```python
from build123d import *

# Parameters (mm, degrees)
F0_W      = 1.1809540468
F0_H      = 55.4866959378
F0_W_2    = 1.0430663562
F0_H_2    = 55.8827305807
F0_W_3    = 1.2505598919
F0_H_3    = 59.9420672474
F1_DEPTH  = 25.4
F2_DEPTH  = 19.05
F4_R      = 25.4
F5_R      = 12.7
F6_DEPTH  = 61.6204
F7_DEPTH  = 45.466
F8_DEPTH  = 87.0204
F10_DEPTH = 37.285599403


with BuildPart() as f1:
    # F0 (on Top) → F1 (new body)
    with BuildSketch(Plane.XY):
        with BuildLine():
            ThreePointArc((-31.4129105711, -45.2980363816), (-30.4781671858, -42.3561098061), (-30.1620009138, -39.2854883608))
            ThreePointArc((-30.1620009138, -39.2854883608), (-29.8463674498, -42.3560514479), (-28.912179671, -45.2980363816))
            Line((-28.912179671, -45.2980363816), (-12.330923231, -45.2980363816))
            Line((-12.330923231, -45.2980363816), (-1.2493222605, -45.2980363816))
            ThreePointArc((-1.2493222605, -45.2980363816), (-0.3153893091, -42.3572770972), (0.0004989823, -39.2879920805))
            Line((0.0004989823, -39.2879920805), (0, -47.9196608067))
            ThreePointArc((0, -47.9196608067), (0.6558623791, -52.3187849866), (2.5664044493, -56.3352857035))
            Line((2.5664044493, -56.3352857035), (27.5960955507, -56.3352857035))
            ThreePointArc((27.5960955507, -56.3352857035), (29.5066376209, -52.3187849866), (30.1625, -47.9196608067))
            Line((30.1625, -47.9196608067), (30.1656608492, -43.188519241))
            ThreePointArc((30.1656608492, -43.188519241), (30.9988064443, -48.131759315), (33.4061909682, -52.5288326332))
            Line((33.4061909682, -52.5288326332), (57.0876307301, -52.5288326332))
            ThreePointArc((57.0876307301, -52.5288326332), (59.4950152541, -48.131759315), (60.3281608492, -43.188519241))
            Line((60.3281608492, -43.188519241), (60.3281608492, 25.6428197026))
            ThreePointArc((60.3281608492, 25.6428197026), (46.2008131527, 40.6938718904), (30.2863311656, 27.5468042333))
            ThreePointArc((30.2863311656, 27.5468042333), (15.0360783361, 42.4746485662), (0, 27.3310989141))
            Line((0, 27.3310989141), (0, 31.4158573747))
            ThreePointArc((0, 31.4158573747), (-15.0810004563, 46.496857831), (-30.1620009126, 31.4158573747))
            Line((-30.1620009126, 31.4158573747), (-30.1620009127, 26.0546095664))
            ThreePointArc((-30.1620009127, 26.0546095664), (-45.243250861, 41.1358595153), (-60.3245008099, 26.0546095669))
            Line((-60.3245008099, 26.0546095669), (-60.3245008099, 0))
            Line((-60.3245008099, 0), (-60.3245008099, -39.2829846411))
            ThreePointArc((-60.3245008099, -39.2829846411), (-60.0085894761, -42.3548841799), (-59.0735911526, -45.2980363816))
            Line((-59.0735911526, -45.2980363816), (-31.4129105711, -45.2980363816))
        make_face()
        with Locations((-30.1620009133, -10.8462562301)):
            Rectangle(F0_W, F0_H, mode=Mode.SUBTRACT)
        with Locations((0.0002494911, -11.0644246154)):
            Rectangle(F0_W_2, F0_H_2, mode=Mode.SUBTRACT)
        with Locations((30.1857188067, -13.1142732591)):
            Rectangle(F0_W_3, F0_H_3, mode=Mode.SUBTRACT)
    extrude(amount=F1_DEPTH)

    # F0 (on Top) → F2 (join)
    with BuildSketch(Plane.XY):
        with BuildLine():
            ThreePointArc((-28.912179671, -45.2980363816), (-29.8463674498, -42.3560514479), (-30.1620009138, -39.2854883608))
            ThreePointArc((-30.1620009138, -39.2854883608), (-30.4781671858, -42.3561098061), (-31.4129105711, -45.2980363816))
            Line((-31.4129105711, -45.2980363816), (-59.0735911526, -45.2980363816))
            ThreePointArc((-59.0735911526, -45.2980363816), (-60.0085894761, -42.3548841799), (-60.3245008099, -39.2829846411))
            Line((-60.3245008099, -39.2829846411), (-60.3245008099, 0))
            Line((-60.3245008099, 0), (-70.1869130135, -37.5586524606))
            Line((-70.1869130135, -37.5586524606), (-70.1869130135, -49.070879817))
            Line((-70.1869130135, -49.070879817), (-63.4611696021, -73.2465684414))
            Line((-63.4611696021, -73.2465684414), (-12.330923231, -73.2465684414))
            ThreePointArc((-12.330923231, -73.2465684414), (1.6433427989, -59.2723024115), (-12.330923231, -45.2980363816))
            Line((-12.330923231, -45.2980363816), (-28.912179671, -45.2980363816))
        make_face()
    extrude(amount=F2_DEPTH)

    # F4
    f4_edges = [f1.edges().sort_by_distance(p)[0] for p in [
        (-70.186913, -37.558652, 9.525),
        (-70.186913, -49.07088, 9.525),
    ]]
    fillet(f4_edges, radius=F4_R)

    # F5
    f5_edges = [f1.edges().sort_by_distance(p)[0] for p in [
        (-63.46117, -73.246568, 9.525),
    ]]
    fillet(f5_edges, radius=F5_R)

    # F3 (on face) → F6 (join)
    with BuildSketch(Plane.XY):
        with BuildLine():
            Line((-30.7524779367, -35.9619690384), (-39.3256613186, -35.9619690384))
            Line((-39.3256613186, -35.9619690384), (-39.3256613186, -42.5913690384))
            Line((-39.3256613186, -42.5913690384), (-30.529074842, -42.5913690384))
            ThreePointArc((-30.529074842, -42.5913690384), (-30.2541193355, -40.9485795087), (-30.1620009138, -39.2854883608))
            ThreePointArc((-30.1620009138, -39.2854883608), (-30.0701620308, -40.9485637633), (-29.7954894935, -42.5913690384))
            Line((-29.7954894935, -42.5913690384), (-0.366012438, -42.5913690384))
            ThreePointArc((-0.366012438, -42.5913690384), (-0.0914778965, -40.9498079941), (0.0004989823, -39.2879920805))
            Line((0.0004989823, -39.2879920805), (0.0003080196, -42.5913690384))
            Line((0.0003080196, -42.5913690384), (29.4575386814, -42.5913690384))
            Line((29.4575386814, -42.5913690384), (29.4575386814, -35.9619690384))
            Line((29.4575386814, -35.9619690384), (0.5217826692, -35.9619690384))
            Line((0.5217826692, -35.9619690384), (0.5217826692, -39.0057899058))
            Line((0.5217826692, -39.0057899058), (-0.5212836869, -39.0057899058))
            Line((-0.5212836869, -39.0057899058), (-0.5212836869, -35.9619690384))
            Line((-0.5212836869, -35.9619690384), (-29.5715238899, -35.9619690384))
            Line((-29.5715238899, -35.9619690384), (-29.5715238899, -38.5896041989))
            Line((-29.5715238899, -38.5896041989), (-30.7524779367, -38.5896041989))
            Line((-30.7524779367, -38.5896041989), (-30.7524779367, -35.9619690384))
        make_face()
    extrude(amount=-F6_DEPTH)

    # F7 (add): a face of the model
    f7_faces = [f1.faces().sort_by_distance(p)[0] for p in [
        (-39.3256613186, -39.2766690384, -30.8102),
    ]]
    extrude(f7_faces, amount=-F7_DEPTH)

    # F8 (add, through all): a face of the model
    f8_faces = [f1.faces().sort_by_distance(p)[0] for p in [
        (-4.9340613186, -39.2766690384, -61.6204),
    ]]
    extrude(f8_faces, amount=-F8_DEPTH)

    # F9 (on face) → F10 (cut, through all)
    with BuildSketch(Plane(origin=(0, -35.9619690384, 0), x_dir=(-1, 0, 0), z_dir=(0, 1, 0))):
        with BuildLine():
            ThreePointArc((-23.3615386814, -50.546), (-25.2030386814, -48.7045), (-27.0445386814, -50.546))
            Line((-27.0445386814, -50.546), (-23.3615386814, -50.546))
        make_face()
        with BuildLine():
            Line((-23.3615386814, -50.546), (-27.0445386814, -50.546))
            ThreePointArc((-27.0445386814, -50.546), (-25.2030386814, -52.3875), (-23.3615386814, -50.546))
        make_face()
        with BuildLine():
            Line((-7.1055386814, -50.546), (-3.4225386814, -50.546))
            ThreePointArc((-3.4225386814, -50.546), (-5.2640386814, -48.7045), (-7.1055386814, -50.546))
        make_face()
        with BuildLine():
            ThreePointArc((-7.1055386814, -50.546), (-5.2640386814, -52.3875), (-3.4225386814, -50.546))
            Line((-3.4225386814, -50.546), (-7.1055386814, -50.546))
        make_face()
        with BuildLine():
            Line((13.2906613186, -50.546), (16.9736613186, -50.546))
            ThreePointArc((16.9736613186, -50.546), (15.1321613186, -48.7045), (13.2906613186, -50.546))
        make_face()
        with BuildLine():
            ThreePointArc((13.2906613186, -50.546), (15.1321613186, -52.3875), (16.9736613186, -50.546))
            Line((16.9736613186, -50.546), (13.2906613186, -50.546))
        make_face()
        with BuildLine():
            Line((33.2296613186, -50.546), (36.9126613186, -50.546))
            ThreePointArc((36.9126613186, -50.546), (35.0711613186, -48.7045), (33.2296613186, -50.546))
        make_face()
        with BuildLine():
            ThreePointArc((33.2296613186, -50.546), (35.0711613186, -52.3875), (36.9126613186, -50.546))
            Line((36.9126613186, -50.546), (33.2296613186, -50.546))
        make_face()
    extrude(amount=-F10_DEPTH, mode=Mode.SUBTRACT)


solid = f1.part
```
Can you work these out from the model? Positions are in its coordinate system, mm. A direction names the side the tool comes from. Coordinates: 2 decimals unless noted, no trailing zeros. Write each loop counter-clockwise with the first axis right and the second up, starting at its lowest first coordinate (ties: lowest second). Pieces come first, ordered by that corner, then holes. Notation, with made-up numbers: (-29.75, 25.25) - (0.25, 25.25) arc R20 ccw to (0.25, 60.25) - close; hole circle Ø11 at (63, 59). An arc over 180 degrees is marked (long way). Return JSON: item names as keys, results as strings.
Q1. If we section it at C-C (x = -23): Please give me the cut outline in (y, z), then the cut area to 3 significant figures.
Computed values:
{"outline": "(-73.25, 0) - (-42.59, 0) - (-42.59, -61.62) - (-35.96, -61.62) - (-35.96, 0) - (44.25, 0) - (44.25, 25.4) - (-45.3, 25.4) - (-45.3, 19.05) - (-73.25, 19.05) - close", "area": "3,220 mm2"}
Q2. If we section it at D-D (z = -26): Please give me the cut outline in (x, y).
Computed values:
{"outline": "(-39.33, -42.59) - (29.46, -42.59) - (29.46, -35.96) - (-39.33, -35.96) - close"}
Q3. On a 3-axis mill with a long thin cutter (end or side, diameter ignored), from which of +Z, -Z, +X, -X, +Y, -Y can I reach the whole of each face in a straight line? I mean faces 3 (the flat face through (30.811, -14, 13)), 4 (the flat face through (-45, -45.298, 22)), 5 (the flat face through (-39.326, -39, -30)). Say none if no direction works.
Computed values:
{"face 3": "+Z, -Z", "face 4": "+Z, -X, -Y", "face 5": "-Z, -X, +Y, -Y"}
Q4. Please list where these lines run through material, in increasing order: L1, parallel to Z at x = -2, y = -63; L2, parallel to Z at x = 29.5, y = -15; L3, parallel to Y at x = 25, z = -38.5. Write a range as from..to.
Computed values:
{"L1": "z = 0..19.05", "L2": "z = 0..25.4", "L3": "y = -42.59..-35.96"}
Q5. I'm going to push flat-ended pins straight in: pin 1 Ø4 at (x, z) = (-15.13, -50.55) entering from -Y; pin 2 Ø1 at (x, y) = (16, -49) entering from -Z; pin 3 Ø3.5 at (y, z) = (28.5, 18) entering from +X. Where does each tip first touch, or does it pass through?
Computed values:
{"pin 1": "stops at y = -42.59", "pin 2": "stops at z = 0", "pin 3": "stops at x = 60.29"}
Q6. If we section it at A-A (y = 13.5): Please give me the cut outline in (x, z).
Computed values:
{"outline": "(-60.32, 0) - (-30.75, 0) - (-30.75, 25.4) - (-60.32, 25.4) - close; (-29.57, 0) - (-0.52, 0) - (-0.52, 25.4) - (-29.57, 25.4) - close; (0.52, 0) - (29.56, 0) - (29.56, 25.4) - (0.52, 25.4) - close; (30.81, 0) - (60.33, 0) - (60.33, 25.4) - (30.81, 25.4) - close"}
Q7. Thinking about a two-plate mould opening in Z: for faces 1 (the cylindrical face through (-14.282, -39.23, -48.912)), 2 (the cylindrical face through (-61.587, -70.589, 9.658)), which applies, +Z half, -Z half, draft (parallel to the pull), parting line (faces both ways), or undercut?
Computed values:
{"face 1": "undercut", "face 2": "draft"}
Q8. If we section it at B-B (y = -25): Please give me the cut outline in (x, z), then the cut area to 3 significant figures.
Computed values:
{"outline": "(-66.89, 0) - (-30.75, 0) - (-30.75, 25.4) - (-60.32, 25.4) - (-60.32, 19.05) - (-66.89, 19.05) - close; (-29.57, 0) - (-0.52, 0) - (-0.52, 25.4) - (-29.57, 25.4) - close; (0.52, 0) - (29.56, 0) - (29.56, 25.4) - (0.52, 25.4) - close; (30.81, 0) - (60.33, 0) - (60.33, 25.4) - (30.81, 25.4) - close", "area": "3,100 mm2"}
